from build123d import *

# Parameters (mm, degrees)
CYLINDER017_R     = 15.8
CYLINDER017_DEPTH = 10
CYLINDER018_R     = 20
CYLINDER018_DEPTH = 10
CYLINDER016_R     = 1.65
CYLINDER016_DEPTH = 50
ARRAY002_Z_COUNT  = 6
ARRAY002_Z_PITCH  = 17
CYLINDER020_R     = 1.65
CYLINDER020_DEPTH = 50
CYLINDER015_R     = 1.65
CYLINDER015_DEPTH = 50
CYLINDER019_R     = 20
CYLINDER019_DEPTH = 10
CYLINDER014_R     = 15.8
CYLINDER014_DEPTH = 115


with BuildPart() as cylinder016:
    # Cylinder017 → Cylinder017 (new body)
    with BuildSketch(Plane.XY):
        Circle(CYLINDER017_R)
    extrude(amount=CYLINDER017_DEPTH)


with BuildPart() as cut012:
    # Cylinder018 → Cylinder018 (new body)
    with BuildSketch(Plane.XY):
        Circle(CYLINDER018_R)
    extrude(amount=CYLINDER018_DEPTH)

    # Cut012: cut Cylinder016
    add(cylinder016.part, mode=Mode.SUBTRACT)


with BuildPart() as cut012_1:
    # Cut012 placement: moved
    add(cut012.part.moved(Location((0, 0, 190.5))))


with BuildPart() as array002:
    # Cylinder016 → Cylinder016 (new body)
    with BuildSketch(Plane(origin=(-25, 0, 15), x_dir=(0, 0, -1), z_dir=(1, 0, 0))):
        Circle(CYLINDER016_R)
    extrude(amount=CYLINDER016_DEPTH)

    # Array002 Z: Array002 ×6


with BuildPart() as array002_1:
    add(array002.part)
    with Locations(*[(0, 0, i * ARRAY002_Z_PITCH) for i in range(1, ARRAY002_Z_COUNT)]):
        add(array002.part)


with BuildPart() as array002_2:
    # Array002 placement: moved
    add(array002_1.part.moved(Location((0, 0, 85))))


with BuildPart() as cylinder020:
    # Cylinder020 → Cylinder020 (new body)
    with BuildSketch(Plane(origin=(-25, 0, 15), x_dir=(0, 0, -1), z_dir=(1, 0, 0))):
        Circle(CYLINDER020_R)
    extrude(amount=CYLINDER020_DEPTH)


with BuildPart() as cylinder013:
    # Cylinder015 → Cylinder015 (new body)
    with BuildSketch(Plane(origin=(-25, 0, 100), x_dir=(0, 0, -1), z_dir=(1, 0, 0))):
        Circle(CYLINDER015_R)
    extrude(amount=CYLINDER015_DEPTH)


with BuildPart() as cylinder019:
    # Cylinder019 → Cylinder019 (new body)
    with BuildSketch(Plane.XY.offset(115)):
        Circle(CYLINDER019_R)
    extrude(amount=CYLINDER019_DEPTH)


with BuildPart() as cut011:
    # Cylinder014 → Cylinder014 (new body)
    with BuildSketch(Plane.XY):
        Circle(CYLINDER014_R)
    extrude(amount=CYLINDER014_DEPTH)

    # Fusion002: union Cylinder019
    add(cylinder019.part)

    # Cut013: cut Cylinder013
    add(cylinder013.part, mode=Mode.SUBTRACT)

    # Cut014: cut Cylinder020
    add(cylinder020.part, mode=Mode.SUBTRACT)


with BuildPart() as cut011_1:
    # Cut014 placement: moved
    add(cut011.part.moved(Location((0, 0, 85))))

    # Cut010: cut Array002
    add(array002_2.part, mode=Mode.SUBTRACT)

    # Cut011: cut Cut012
    add(cut012_1.part, mode=Mode.SUBTRACT)


solid = cut011_1.part
Input: part model. Units: mm. Frame: model coordinates. A direction names the side the tool comes from. Coordinates: 2 decimals unless noted, no trailing zeros. Order: outer loops, then holes, each group sorted by start corner. A loop starts at its lowest first (then second) coordinate and runs counter-clockwise, first axis right, second up. Notation, with made-up numbers: M 33.25,5.5 L 72.25,5.5 A20 ccw 72.25,27.5 Z; hole C 8.5,64 d4. An arc over 180 degrees is marked long. Answer as CSV lines item,"result".
1. Material intervals for line 1 (Y direction, x = -0.5, z = 151); line 2 (Z direction, x = 16, y = -9.5); line 3 (Y direction, x = 7.5, z = 185), sorted ascending. Write a range as from..to.
Reported:
line 1,"-15.79..-1.65, 1.65..15.79"
line 2,"200.5..210"
line 3,"-13.91..-1.65, 1.65..13.91"
2. Section C-C (z = 185). Return the cut outline in (x, y), then the cut area to 3 significant figures.
Reported:
outline,"M -15.71,-1.65 A15.8 ccw 15.71,-1.65 Z; M -15.71,1.65 L 15.71,1.65 A15.8 ccw Z"
area,"680 mm2"
3. Section D-D (x = 12). Return the cut outline in (y, z), then the cut area to 3 significant figures.
Reported:
outline,"M -16,200.5 L -10.28,200.5 L -10.28,85 L 10.28,85 L 10.28,200.5 L 16,200.5 L 16,210 L -16,210 Z; hole C 0,100 d3.3; hole C 0,117 d3.3; hole C 0,134 d3.3; hole C 0,151 d3.3; hole C 0,168 d3.3; hole C 0,185 d3.3"
area,"2,630 mm2"
4. Pull-direction query (Z, two-part tool) for faces 3 (the cylindrical face through (-0.222, -0.632, 132.476)), 4 (the flat face through (0, 0, 210)), 5 (the flat face through (15, 6, 200.5)), 6 (the cylindrical face through (-0.222, -0.632, 166.476)); classes: released by +Z, released by -Z, zero draft, split by the parting line, or undercut.
Reported:
face 3,"undercut"
face 4,"released by +Z"
face 5,"released by -Z"
face 6,"undercut"
5. First-contact query: P1, Ø5, axis at y = 8, z = 194, coming from the +X side; P2, Ø2, axis at x = -0.5, z = 98.5, coming from the +Y side; P3, Ø6, axis at y = 8, z = 133.5, coming from the +X side; P4, Ø3, axis at y = 0, z = 168, coming from the -X side. Flat tips, straight axial feed; report the tip coordinate or a pass-through.
Reported:
P1,"x = 14.81"
P2,"y = 15.8"
P3,"x = 14.99"
P4,"through"
6. Access query for faces 1 (the cylindrical face through (15.07, 4.75, 141.94)), 2 (the cylindrical face through (-0.222, -0.632, 183.476)). Directions: +Z, -Z, +X, -X, +Y, -Y. A direction counts if a zero-diameter tool reaches every point of the face in a straight line with its end or side. Return the directions, or none.
Reported:
face 1,"-Z"
face 2,"+X, -X"
7. Section A-A (x = 0). Return the cut outline in (y, z), then the cut area to 3 significant figures.
Reported:
outline,"M -20,200.5 L -15.8,200.5 L -15.8,85 L 15.8,85 L 15.8,200.5 L 20,200.5 L 20,210 L -20,210 Z; hole C 0,100 d3.3; hole C 0,117 d3.3; hole C 0,134 d3.3; hole C 0,151 d3.3; hole C 0,168 d3.3; hole C 0,185 d3.3"
area,"3,980 mm2"
8. Section B-B (y = -12.5). Return the cut outline in (x, z), then the cut area to 3 significant figures.
Reported:
outline,"M -15.61,200.5 L -9.66,200.5 L -9.66,85 L 9.66,85 L 9.66,200.5 L 15.61,200.5 L 15.61,210 L -15.61,210 Z"
area,"2,530 mm2"
